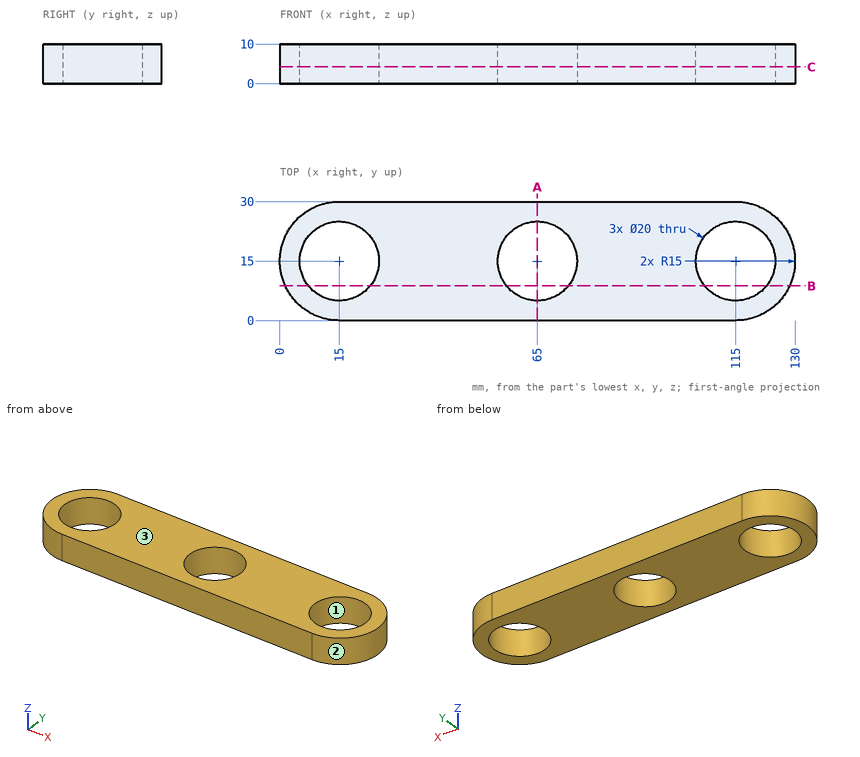
For this review, use the dimensioned drawing (mm, ordinates from the lowest corner) and the shaded views. Coordinates: 2 decimals unless noted, no trailing zeros. Write each loop counter-clockwise with the first axis right and the second up, starting at its lowest first coordinate (ties: lowest second). Pieces come first, ordered by that corner, then holes. Notation, with made-up numbers: (-31, 55) -> (3, 55) arc R21 ccw to (3, 81) -> close; hole circle Ø6 at (82.5, 8). An arc over 180 degrees is marked (long way). Put each result on its own line as item: value.
Q1. Wall thickness on L1, parallel to Y at x = 65, z = 6; L2, parallel to X at y = 12, z = 3; L3, parallel to X at y = 8.5, z = 5: over which ranges is each line inside the solid? List them lowest first.
From the geometry:
L1: y = 0 to 5, 25 to 30
L2: x = 0.3 to 5.46, 24.54 to 55.46, 74.54 to 105.46, 124.54 to 129.7
L3: x = 1.48 to 7.4, 22.6 to 57.4, 72.6 to 107.4, 122.6 to 128.52
Q2. Take a section at A-A, the plane x = 65. State the section outline as (y, z) points, then the cut area to 3 significant figures.
From the geometry:
outline: (0, 0) -> (5, 0) -> (5, 10) -> (0, 10) -> close; (25, 0) -> (30, 0) -> (30, 10) -> (25, 10) -> close
area: 100 mm2
Q3. Take a section at B-B, the plane y = 8.75. State the section outline as (x, z) points, then the cut area to 3 significant figures.
From the geometry:
outline: (1.36, 0) -> (7.19, 0) -> (7.19, 10) -> (1.36, 10) -> close; (22.81, 0) -> (57.19, 0) -> (57.19, 10) -> (22.81, 10) -> close; (72.81, 0) -> (107.19, 0) -> (107.19, 10) -> (72.81, 10) -> close; (122.81, 0) -> (128.64, 0) -> (128.64, 10) -> (122.81, 10) -> close
area: 804 mm2
Q4. The part is to be moulded in two halves that separate along X. For the marked faces 1, 2 and 3, say which applies: +X half, -X half, draft (parallel to the pull), parting line (faces both ways), or undercut.
From the geometry:
face 1: undercut
face 2: +X half
face 3: draft
Q5. Take a section at C-C, the plane z = 4.25. State the section outline as (x, y) points, then the cut area to 3 significant figures.
From the geometry:
outline: (15, 0) -> (115, 0) arc R15 ccw to (115, 30) -> (15, 30) arc R15 ccw to start; hole circle Ø20 at (15, 15); hole circle Ø20 at (65, 15); hole circle Ø20 at (115, 15)
area: 2,760 mm2
Q6. Clearance check with flat-ended pins moving along their axes: pin 1 Ø10 at (x, y) = (113, 20) entering from -Z; pin 2 Ø6 at (y, z) = (4, 6) entering from +X; pin 3 Ø2 at (y, z) = (13, 3) entering from +X. State where each tip first meets the part, or that it passes through.
From the geometry:
pin 1: stops at z = 0
pin 2: stops at x = 127.69
pin 3: stops at x = 129.97
